```python
from build123d import *

# Parameters (mm, degrees)
TABAN_FLAN_1_DEPTH    = 25
IZIM9_W               = 9.15
IZIM9_H               = 8
IZIM9_H_2             = 19
KES_EKSTR_ZYON1_DEPTH = 32.162677998
IZIM11_R              = 2.6
KES_EKSTR_ZYON2_DEPTH = 10
RADYUS1_R             = 2.5


# Sheet-metal steps are written as plain solids
with BuildPart() as part:
    # Çizim1 → Taban-Flanş1 (new, symmetric)
    with BuildSketch(Plane.XY):
        with BuildLine():
            Line((-12.5, 0), (12.5, 0))
            ThreePointArc((12.5, 0), (14.537154879, -7.765591238), (8.95035213, -2))
            Line((8.95035213, -2), (10.233357384, -2.777108434))
            ThreePointArc((10.233357384, -2.777108434), (13.800833838, -6.458751031), (12.5, -1.5))
            Line((12.5, -1.5), (-12.5, -1.5))
            Line((-12.5, -1.5), (-12.5, 0))
        make_face()
    extrude(amount=TABAN_FLAN_1_DEPTH, both=True)

    # Çizim9 → Kes-Ekstrüzyon1 (cut, through all)
    with BuildSketch(Plane(origin=(0, 0, 0), x_dir=(1, 0, 0), z_dir=(0, 1, 0))):
        with Locations((12.075, 21)):
            Rectangle(IZIM9_W, IZIM9_H)
        with Locations((12.075, -21)):
            Rectangle(IZIM9_W, IZIM9_H)
        with Locations((12.075, 0)):
            Rectangle(IZIM9_W, IZIM9_H_2)
    extrude(amount=-KES_EKSTR_ZYON1_DEPTH, mode=Mode.SUBTRACT)

    # Çizim11 → Kes-Ekstrüzyon2 (cut)
    with BuildSketch(Plane(origin=(0, 0, 0), x_dir=(1, 0, 0), z_dir=(0, 1, 0))):
        with Locations(Location((-2.5, 15, 0), (0, 0, 180))):
            Circle(IZIM11_R)
        with Locations(Location((-2.5, -15, 0), (0, 0, 180))):
            Circle(IZIM11_R)
    extrude(amount=-KES_EKSTR_ZYON2_DEPTH, mode=Mode.SUBTRACT)

    # Radyus1
    radyus1_edges = [part.edges().sort_by_distance(p)[0] for p in [
        (-12.5, -0.75, 25),
        (-12.5, -0.75, -25),
    ]]
    fillet(radyus1_edges, radius=RADYUS1_R)


solid = part.part
```
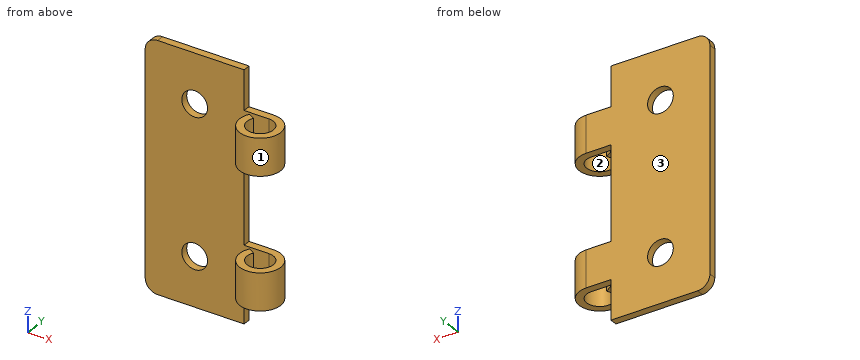
Input: part model. Units: mm. Frame: model coordinates. Face numbers are marked on the shaded views. Give positions to 0.01 mm unless a question says otherwise; leave off trailing zeros. Order: outer loops, then holes, each group sorted by start corner. A loop starts at its lowest first (then second) coordinate and runs counter-clockwise, first axis right, second up.
1. Cut plane C-C (z = -15). Return loops of the section in (x, y).
Computed:
outline: (-12.5, -1.5) - (-5.1, -1.5) - (-5.1, 0) - (-12.5, 0) - close; (0.1, -1.5) - (12.5, -1.5) arc R2.65 cw (long way) to (10.23, -2.78) - (8.95, -2) arc R4.15 ccw (long way) to (12.5, 0) - (0.1, 0) - close
2. Pin query (flat end, axial travel): pin 1 Ø4 at (x, y) = (12.5, -4.15) entering from +Z; pin 2 Ø7 at (x, z) = (-2.5, -15) entering from -Y; pin 3 Ø4 at (x, y) = (12, -5) entering from -Z; pin 4 Ø0.8 at (y, z) = (-1, -3.5) entering from +X. Return the tip coordinate at first contact, or that it passes through.
Computed:
pin 1: passes through
pin 2: stops at y = -1.5
pin 3: stops at z = -17
pin 4: stops at x = 7.5
3. Line query: probe 1 along Z at (x, y) = (-2.5, -1.1); probe 2 along X at (y, z) = (-4.15, 14); probe 3 along Y at (x, z) = (12.5, 12). Output: solid intervals per line, ascending.
Computed:
probe 1: z = -25 to -17.6, -12.4 to 12.4, 17.6 to 25
probe 2: x = 8.35 to 9.85, 15.15 to 16.65
probe 3: y = -8.3 to -6.8, -1.5 to 0
4. Cut plane A-A (x = -2.5). Return loops of the section in (y, z).
Computed:
outline: (-1.5, -25) - (0, -25) - (0, -17.6) - (-1.5, -17.6) - close; (-1.5, -12.4) - (0, -12.4) - (0, 12.4) - (-1.5, 12.4) - close; (-1.5, 17.6) - (0, 17.6) - (0, 25) - (-1.5, 25) - close
5. Draft query along X for the marked faces 1, 2 and 3. Return one class per face: released by +X, released by -X, zero draft, split by the parting line, or undercut.
Computed:
face 1: split by the parting line
face 2: undercut
face 3: zero draft
6. Cut plane B-B (y = -4.15). Return loops of the section in (x, z), and give its area (3 significant figures).
Computed:
outline: (8.35, -17) - (9.85, -17) - (9.85, -9.5) - (8.35, -9.5) - close; (8.35, 9.5) - (9.85, 9.5) - (9.85, 17) - (8.35, 17) - close; (15.15, -17) - (16.65, -17) - (16.65, -9.5) - (15.15, -9.5) - close; (15.15, 9.5) - (16.65, 9.5) - (16.65, 17) - (15.15, 17) - close
area: 45.0 mm2
7. Cut plane D-D (y = -0.75). Return loops of the section in (x, z), and give its area (3 significant figures).
Computed:
outline: (-12.5, -22.5) arc R2.5 ccw to (-10, -25) - (7.5, -25) - (7.5, -17) - (14.88, -17) - (14.88, -9.5) - (7.5, -9.5) - (7.5, 9.5) - (14.88, 9.5) - (14.88, 17) - (7.5, 17) - (7.5, 25) - (-10, 25) arc R2.5 ccw to (-12.5, 22.5) - close; hole circle Ø5.2 at (-2.5, -15); hole circle Ø5.2 at (-2.5, 15)
area: 1,070 mm2
